Geometry check sheet. Reference: the model listing, model coordinates, mm. A direction names the side the tool comes from. Coordinates: 2 decimals unless noted, no trailing zeros. Write each loop counter-clockwise with the first axis right and the second up, starting at its lowest first coordinate (ties: lowest second). Pieces come first, ordered by that corner, then holes. Notation, with made-up numbers: M 52,-15 L 69,-15 A20 ccw 69,8 Z; hole C 10.5,40.25 d3. An arc over 180 degrees is marked long. Answer as a JSON object with one key per item and string values. Group by question number.
```python
from build123d import *

# Parameters (mm, degrees)
SKETCH1_W           = 70
SKETCH1_H           = 55
BOSS_EXTRUDE1_DEPTH = 5
SKETCH2_W           = 5
SKETCH2_H           = 45
SKETCH2_W_2         = 5.019591865
CUT_EXTRUDE1_DEPTH  = 5
BOSS_EXTRUDE4_DEPTH = 50
SKETCH7_W           = 42.1
SKETCH7_H           = 42.1
CUT_EXTRUDE2_DEPTH  = 5
SKETCH9_W           = 5
SKETCH9_H           = 10
BOSS_EXTRUDE5_DEPTH = 5
SKETCH11_W          = 5
SKETCH11_H          = 10
BOSS_EXTRUDE6_DEPTH = 5


with BuildPart() as part:
    # Sketch1 → Boss-Extrude1 (new body)
    with BuildSketch(Plane.XY):
        with Locations((-35, 27.5)):
            Rectangle(SKETCH1_W, SKETCH1_H)
    extrude(amount=BOSS_EXTRUDE1_DEPTH)

    # Sketch2 → Cut-Extrude1 (cut)
    with BuildSketch(Plane.XY.offset(5)):
        with Locations((-62.5, 27.5)):
            Rectangle(SKETCH2_W, SKETCH2_H)
        with Locations((-7.509795933, 27.5)):
            Rectangle(SKETCH2_W_2, SKETCH2_H)
    extrude(amount=-CUT_EXTRUDE1_DEPTH, mode=Mode.SUBTRACT)

    # Sketch6 → Boss-Extrude4 (add)
    with BuildSketch(Plane.XY.offset(5)):
        Polygon((-70, 0), (-65, 0), (-65, 50), (-5, 50), (-5, 0), (0, 0), (0, 55), (-5, 55), (-65, 55), (-70, 55), align=None)
    extrude(amount=BOSS_EXTRUDE4_DEPTH)

    # Sketch7 → Cut-Extrude2 (cut)
    with BuildSketch(Plane(origin=(0, 55, 0), x_dir=(1, 0, 0), z_dir=(0, 1, 0))):
        with Locations((-35, -33.95)):
            Rectangle(SKETCH7_W, SKETCH7_H)
    extrude(amount=-CUT_EXTRUDE2_DEPTH, mode=Mode.SUBTRACT)

    # Sketch9 → Boss-Extrude5 (add)
    with BuildSketch(Plane.ZY.offset(60)):
        with Locations((2.5, 45)):
            Rectangle(SKETCH9_W, SKETCH9_H)
    extrude(amount=BOSS_EXTRUDE5_DEPTH)

    # Sketch11 → Boss-Extrude6 (add)
    with BuildSketch(Plane(origin=(-10.019591865, 0, 0), x_dir=(0, 0, -1), z_dir=(1, 0, 0))):
        with Locations((-2.5, 45)):
            Rectangle(SKETCH11_W, SKETCH11_H)
    extrude(amount=BOSS_EXTRUDE6_DEPTH)


solid = part.part
```
1) Section check B-B (z = 40). Record the cut outline in (x, y).
2) Section check D-D (z = 4). State how many separate pieces and enclosed holes the cut face has, then the cut area to 3 significant figures.
3) Go/stop test with flat-tipped pins: pin 1 Ø5 at (x, y) = (-19, 33) entering from +Z; pin 2 Ø5.5 at (x, y) = (-33, 51.5) entering from +Z; pin 3 Ø10 at (x, z) = (-40.5, 20.5) entering from +Y; pin 4 Ø16.5 at (x, z) = (-21, 26) entering from -Y. Record where each tip stops, or that it passes through.
4) Material ranges on probe 1 along X at (y, z) = (24.5, 3); probe 2 along X at (y, z) = (27.5, 11.5); probe 3 along Y at (x, z) = (-9, 28), recorded low to high. Write a range as [from, to].
5) Section check A-A (y = 36). Record the cut outline in (x, z).
6) Set-up check for faces 5 (the flat face through (-56.05, 53, 34)), 6 (the flat face through (-60, 22, 3)), 7 (the flat face through (-35, 25, 5)): record each of +Z, -Z, +X, -X, +Y, -Y from which the full face is reachable in a straight line by a thin tool's end or side.
7) Draft check along Y on faces 1 (the flat face through (-63, 5, 3)), 2 (the flat face through (-70, 28, 27)), 3 (the flat face through (-35, 55, 9)), 4 (the flat face through (-8, 40, 3)). Enter one of: +Y half, -Y half, draft (parallel to the pull), parting line (faces both ways), or undercut.
8) Section check C-C (y = 43). Record the cut outline in (x, z).
Entries:
{
 "1": {"outline": "M -70,0 L -65,0 L -65,50 L -56.05,50 L -56.05,55 L -70,55 Z; M -13.95,50 L -5,50 L -5,0 L 0,0 L 0,55 L -13.95,55 Z"},
 "2": {"separate pieces": "1", "enclosed holes": "2", "area": "3,500 mm^2"},
 "3": {"pin 1": "z = 5", "pin 2": "z = 12.9", "pin 3": "through", "pin 4": "y = 50"},
 "4": {"probe 1": "[-70, -65], [-60, -10.02], [-5, 0]", "probe 2": "[-70, -65], [-5, 0]", "probe 3": "[50, 55]"},
 "5": {"outline": "M -70,0 L -65,0 L -65,55 L -70,55 Z; M -60,0 L -10.02,0 L -10.02,5 L -60,5 Z; M -5,0 L 0,0 L 0,55 L -5,55 Z"},
 "6": {"face 5": "+Z, +Y, -Y", "face 6": "+Z, -Z", "face 7": "+Z, -Y"},
 "7": {"face 1": "undercut", "face 2": "draft", "face 3": "+Y half", "face 4": "undercut"},
 "8": {"outline": "M -70,0 L -5.02,0 L -5.02,5 L -65,5 L -65,55 L -70,55 Z; M -5,0 L 0,0 L 0,55 L -5,55 Z"}
}
